Source: CAD feature listing. Evaluate the final solid. Frame: model axes, mm. Face numbers are marked on the shaded views. Round coordinates to 2 decimals unless told otherwise and drop trailing zeros. Write each loop counter-clockwise with the first axis right and the second up, starting at its lowest first coordinate (ties: lowest second). Pieces come first, ordered by that corner, then holes.
from build123d import *

# Parameters (mm, degrees)
SKETCH_1_W          = 107
SKETCH_1_H          = 94.5
EXTRUDE_1_DEPTH     = 37
SHELL_1_T           = -2
SKETCH_2_W          = 5
SKETCH_2_H          = 72.15042502
CUT_EXTRUDE_3_DEPTH = 20
SKETCH_6_W          = 5
SKETCH_6_H          = 27
CUT_EXTRUDE_4_DEPTH = 1000


with BuildPart() as part:
    # 草图1 → 凸台-拉伸1 (new body)
    with BuildSketch(Plane(origin=(0, 0, 0), x_dir=(1, 0, 0), z_dir=(0, 1, 0))):
        with Locations((53.5, 47.25)):
            Rectangle(SKETCH_1_W, SKETCH_1_H)
    extrude(amount=EXTRUDE_1_DEPTH)

    # 抽壳1
    shell_1_openings = [part.faces().sort_by_distance(p)[0] for p in [
        (53.5, 18.5, 0),
    ]]
    offset(amount=SHELL_1_T, openings=shell_1_openings, kind=Kind.INTERSECTION)

    # 草图2 → 切除-拉伸3 (cut)
    with BuildSketch(Plane(origin=(0, 37, 0), x_dir=(1, 0, 0), z_dir=(0, 1, 0))):
        with Locations((22.5, 48.42478749)):
            Rectangle(SKETCH_2_W, SKETCH_2_H)
        with Locations((32.5, 48.42478749)):
            Rectangle(SKETCH_2_W, SKETCH_2_H)
        with Locations((42.5, 48.42478749)):
            Rectangle(SKETCH_2_W, SKETCH_2_H)
        with Locations((52.5, 48.42478749)):
            Rectangle(SKETCH_2_W, SKETCH_2_H)
        with Locations((62.5, 48.42478749)):
            Rectangle(SKETCH_2_W, SKETCH_2_H)
        with Locations((72.5, 48.42478749)):
            Rectangle(SKETCH_2_W, SKETCH_2_H)
        with Locations((82.5, 48.42478749)):
            Rectangle(SKETCH_2_W, SKETCH_2_H)
    extrude(amount=-CUT_EXTRUDE_3_DEPTH, mode=Mode.SUBTRACT)

    # 草图6 → 切除-拉伸4 (cut)
    with BuildSketch(Plane.ZY):
        with Locations((-82, 18.5)):
            Rectangle(SKETCH_6_W, SKETCH_6_H)
        with Locations((-72, 18.5)):
            Rectangle(SKETCH_6_W, SKETCH_6_H)
        with Locations((-62, 18.5)):
            Rectangle(SKETCH_6_W, SKETCH_6_H)
        with Locations((-52, 18.5)):
            Rectangle(SKETCH_6_W, SKETCH_6_H)
        with Locations((-42, 18.5)):
            Rectangle(SKETCH_6_W, SKETCH_6_H)
        with Locations((-32, 18.5)):
            Rectangle(SKETCH_6_W, SKETCH_6_H)
        with Locations((-22, 18.5)):
            Rectangle(SKETCH_6_W, SKETCH_6_H)
        with Locations((-12, 18.5)):
            Rectangle(SKETCH_6_W, SKETCH_6_H)
    extrude(amount=-CUT_EXTRUDE_4_DEPTH, mode=Mode.SUBTRACT)


solid = part.part
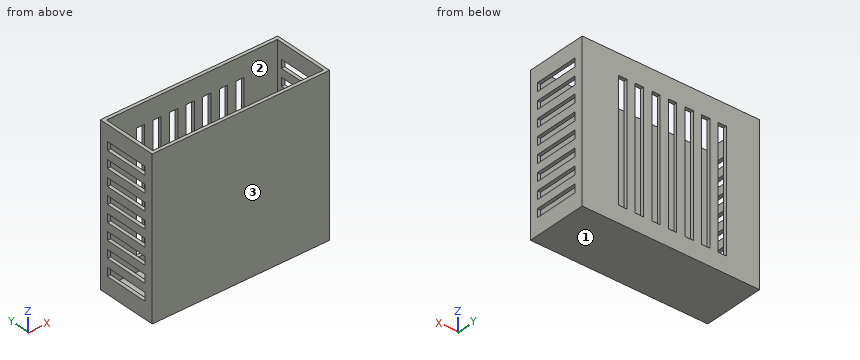
1) Section query A-A on x = 82.5. Return the cut outline in (y, z), then the cut area to 3 significant figures.
Taken from the geometry:
outline: (0, -94.5) - (37, -94.5) - (37, -84.5) - (35, -84.5) - (35, -92.5) - (2, -92.5) - (2, 0) - (0, 0) - close; (35, -12.35) - (37, -12.35) - (37, 0) - (35, 0) - close
area: 300 mm2
2) Pull-direction query (Y, two-part tool) for the marked faces 1, 2 and 3; classes: released by +Y, released by -Y, zero draft, split by the parting line, or undercut.
Taken from the geometry:
face 1: zero draft
face 2: undercut
face 3: released by -Y
3) Contact query for flat-ended pins moving along their axis: P1, Ø3, axis at x = 82, z = -68.5, coming from the -Y side; P2, Ø12, axis at x = 49.5, y = 18.5, coming from the +Z side. Output: stop coordinate, or through.
Taken from the geometry:
P1: stops at y = 0
P2: stops at z = -92.5
4) Material intervals for line 1 (Y direction, x = 90.5, z = -63); line 2 (X direction, y = 18, z = -89.5); line 3 (Z direction, x = 20, y = 28.5), sorted ascending.
Taken from the geometry:
line 1: y = 0 to 2, 35 to 37
line 2: x = 0 to 2, 105 to 107
line 3: z = -94.5 to -92.5
5) Section query B-B on z = -46. State how many separate pieces and enclosed holes the cut face has, then the cut area to 3 significant figures.
Taken from the geometry:
separate pieces: 7
enclosed holes: 0
area: 490 mm2
6) Section query C-C on x = 101. Return the cut outline in (y, z).
Taken from the geometry:
outline: (0, -94.5) - (37, -94.5) - (37, 0) - (35, 0) - (35, -92.5) - (2, -92.5) - (2, 0) - (0, 0) - close
